Part model, mm, in its own coordinate system. Face numbers are marked on the shaded views. A direction names the side the tool comes from. Round coordinates to 2 decimals unless told otherwise and drop trailing zeros. Loops run counter-clockwise (first coordinate to the right, second up) from the corner with the lowest first, then second, coordinate; pieces in that order, holes last. Notation, with made-up numbers: (57.5, 79) - (97.5, 79) arc R31 cw to (97.5, 109) - close; hole circle Ø1 at (-23, 20.25). An arc over 180 degrees is marked (long way). Put each result on its own line as item: value.
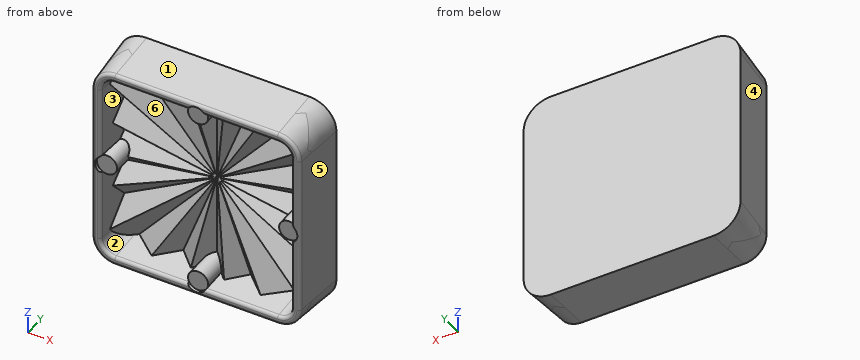
from build123d import *

# Parameters (mm, degrees)
BOSS_EXTRUDE1_DEPTH = 6.35
BOSS_EXTRUDE1_DRAFT = -5
CUT_EXTRUDE3_DEPTH  = 20.05
CIRPATTERN3_COUNT   = 18
BOSS_EXTRUDE3_DEPTH = 6.35
BOSS_EXTRUDE3_DRAFT = -5
FILLET2_R           = 0.381
BOSS_EXTRUDE4_REACH = 20.926
SKETCH8_R           = 1.1811
SKETCH9_R           = 1.1811
CUT_EXTRUDE4_DEPTH  = 19.926409089
CIRPATTERN4_COUNT   = 4


with BuildPart() as part:
    # Sketch1 → Boss-Extrude1 (with draft: the straight prism first)
    with BuildSketch(Plane(origin=(0, 0, 0), x_dir=(1, 0, 0), z_dir=(0, 1, 0))):
        with BuildLine():
            Line((-9.525, -12.7), (9.525, -12.7))
            ThreePointArc((9.525, -12.7), (11.77006403, -11.77006403), (12.7, -9.525))
            Line((12.7, -9.525), (12.7, 9.525))
            ThreePointArc((12.7, 9.525), (11.77006403, 11.77006403), (9.525, 12.7))
            Line((9.525, 12.7), (-9.525, 12.7))
            ThreePointArc((-9.525, 12.7), (-11.77006403, 11.77006403), (-12.7, 9.525))
            Line((-12.7, 9.525), (-12.7, -9.525))
            ThreePointArc((-12.7, -9.525), (-11.77006403, -11.77006403), (-9.525, -12.7))
        make_face()
    extrude(amount=-BOSS_EXTRUDE1_DEPTH)
    # Boss-Extrude1: the draft: its side faces are tilted about the plane it starts from
    boss_extrude1_sides = [part.faces().sort_by_distance(p)[0] for p in [
        (0, -3.175, 12.7),
        (11.77006403, -3.175, 11.77006403),
        (12.7, -3.175, 0),
        (11.77006403, -3.175, -11.77006403),
        (0, -3.175, -12.7),
        (-11.77006403, -3.175, -11.77006403),
        (-12.7, -3.175, 0),
        (-11.77006403, -3.175, 11.77006403),
    ]]
    draft(boss_extrude1_sides, Plane(origin=(0, 0, 0), x_dir=(1, 0, 0), z_dir=(0, 1, 0)), BOSS_EXTRUDE1_DRAFT)

    # Sketch6 → Cut-Extrude3 (cut, through all)
    with BuildSketch(Plane.XY):
        Polygon((0, -2.159), (-7.366, -9.525), (7.366, -9.525), align=None)
    cut_extrude3 = extrude(amount=-CUT_EXTRUDE3_DEPTH, mode=Mode.SUBTRACT)

    # CirPattern3: Cut-Extrude3 ×18 about axis
    cirpattern3_axis = Axis((0, 0, 0), (0, 1, 0))
    for i in range(1, CIRPATTERN3_COUNT):
        add(cut_extrude3.rotate(cirpattern3_axis, i * 360 / CIRPATTERN3_COUNT), mode=Mode.SUBTRACT)


with BuildPart() as boss_extrude3_tool:
    # Sketch7 → Boss-Extrude3 (with draft: the straight prism first)
    with BuildSketch(Plane(origin=(0, 0, 0), x_dir=(1, 0, 0), z_dir=(0, 1, 0))):
        with BuildLine():
            Line((-9.525, -12.7), (9.525, -12.7))
            ThreePointArc((9.525, -12.7), (11.77006403, -11.77006403), (12.7, -9.525))
            Line((12.7, -9.525), (12.7, 9.525))
            ThreePointArc((12.7, 9.525), (11.77006403, 11.77006403), (9.525, 12.7))
            Line((9.525, 12.7), (-9.525, 12.7))
            ThreePointArc((-9.525, 12.7), (-11.77006403, 11.77006403), (-12.7, 9.525))
            Line((-12.7, 9.525), (-12.7, -9.525))
            ThreePointArc((-12.7, -9.525), (-11.77006403, -11.77006403), (-9.525, -12.7))
        make_face()
        with BuildLine():
            Line((-9.525, -10.668), (9.525, -10.668))
            ThreePointArc((9.525, -10.668), (10.333223051, -10.333223051), (10.668, -9.525))
            Line((10.668, -9.525), (10.668, 9.525))
            ThreePointArc((10.668, 9.525), (10.333223051, 10.333223051), (9.525, 10.668))
            Line((9.525, 10.668), (-9.525, 10.668))
            ThreePointArc((-9.525, 10.668), (-10.333223051, 10.333223051), (-10.668, 9.525))
            Line((-10.668, 9.525), (-10.668, -9.525))
            ThreePointArc((-10.668, -9.525), (-10.333223051, -10.333223051), (-9.525, -10.668))
        make_face(mode=Mode.SUBTRACT)
    extrude(amount=-BOSS_EXTRUDE3_DEPTH)
    # Boss-Extrude3: the draft: its side faces are tilted about the plane it starts from
    boss_extrude3_sides = [boss_extrude3_tool.faces().sort_by_distance(p)[0] for p in [
        (0, -3.175, 12.7),
        (11.77006403, -3.175, 11.77006403),
        (12.7, -3.175, 0),
        (11.77006403, -3.175, -11.77006403),
        (0, -3.175, -12.7),
        (-11.77006403, -3.175, -11.77006403),
        (-12.7, -3.175, 0),
        (-11.77006403, -3.175, 11.77006403),
        (-10.333223051, -3.175, 10.333223051),
        (-10.668, -3.175, 0),
        (-10.333223051, -3.175, -10.333223051),
        (0, -3.175, -10.668),
        (10.333223051, -3.175, -10.333223051),
        (10.668, -3.175, 0),
        (10.333223051, -3.175, 10.333223051),
        (0, -3.175, 10.668),
    ]]
    draft(boss_extrude3_sides, Plane(origin=(0, 0, 0), x_dir=(1, 0, 0), z_dir=(0, 1, 0)), BOSS_EXTRUDE3_DRAFT)


with BuildPart() as part_1:
    add(part.part)

    # Boss-Extrude3: add boss_extrude3_tool
    add(boss_extrude3_tool.part)

    # Fillet2
    fillet2_edges = [part_1.edges().sort_by_distance(p)[0] for p in [
        (-11.377228727, -6.35, -11.377228727),
        (-11.377228727, -6.35, 11.377228727),
        (-12.144446987, -6.35, 0),
        (0, -6.35, 12.144446987),
        (11.377228727, -6.35, 11.377228727),
        (12.144446987, -6.35, 0),
        (11.377228727, -6.35, -11.377228727),
        (0, -6.35, -12.144446987),
        (-11.223553013, -6.35, 0),
        (-10.726058354, -6.35, 10.726058354),
        (0, -6.35, 11.223553013),
        (10.726058354, -6.35, 10.726058354),
        (11.223553013, -6.35, 0),
        (10.726058354, -6.35, -10.726058354),
        (0, -6.35, -11.223553013),
        (-10.726058354, -6.35, -10.726058354),
    ]]
    fillet(fillet2_edges, radius=FILLET2_R)

    # Sketch8 → Boss-Extrude4 (add, up to next)
    with BuildSketch(Plane(origin=(0, -5.969, 0), x_dir=(-1, 0, 0), z_dir=(0, -1, 0)), mode=Mode.PRIVATE) as boss_extrude4_sk1:
        with Locations((0, 10.668)):
            Circle(SKETCH8_R)
    boss_extrude4_tool1 = extrude(boss_extrude4_sk1.sketch, amount=-BOSS_EXTRUDE4_REACH, mode=Mode.PRIVATE) - part_1.part
    boss_extrude4 = boss_extrude4_tool1.solids().sort_by_distance((0, -5.969, -10.668))[0]
    add(boss_extrude4)

    # Sketch9 → Cut-Extrude4 (cut, through all)
    with BuildSketch(Plane.XZ.offset(5.969)):
        with Locations((0, -10.668)):
            Circle(SKETCH9_R)
    cut_extrude4 = extrude(amount=CUT_EXTRUDE4_DEPTH, mode=Mode.SUBTRACT)

    # CirPattern4: Boss-Extrude4, Cut-Extrude4; each copy of Boss-Extrude4 runs up to whatever stops it at its own place
    cirpattern4_before = part_1.part  # the part as the pattern finds it: every copy runs up to it
    cirpattern4_boss_extrude4_long = extrude(boss_extrude4_sk1.sketch, amount=-BOSS_EXTRUDE4_REACH, mode=Mode.PRIVATE)
    cirpattern4_boss_extrude4_tool = cirpattern4_boss_extrude4_long.rotate(Axis((0, 0, 0), (0, 1, 0)), 1 * 360 / CIRPATTERN4_COUNT) - cirpattern4_before
    add(cirpattern4_boss_extrude4_tool.solids().sort_by_distance((-10.668, -5.969, 0))[0])
    cirpattern4_boss_extrude4_tool = cirpattern4_boss_extrude4_long.rotate(Axis((0, 0, 0), (0, 1, 0)), 2 * 360 / CIRPATTERN4_COUNT) - cirpattern4_before
    add(cirpattern4_boss_extrude4_tool.solids().sort_by_distance((0, -5.969, 10.668))[0])
    cirpattern4_boss_extrude4_tool = cirpattern4_boss_extrude4_long.rotate(Axis((0, 0, 0), (0, 1, 0)), 3 * 360 / CIRPATTERN4_COUNT) - cirpattern4_before
    add(cirpattern4_boss_extrude4_tool.solids().sort_by_distance((10.668, -5.969, 0))[0])
    add(cut_extrude4.rotate(Axis((0, 0, 0), (0, 1, 0)), 1 * 360 / CIRPATTERN4_COUNT), mode=Mode.SUBTRACT)
    add(cut_extrude4.rotate(Axis((0, 0, 0), (0, 1, 0)), 2 * 360 / CIRPATTERN4_COUNT), mode=Mode.SUBTRACT)
    add(cut_extrude4.rotate(Axis((0, 0, 0), (0, 1, 0)), 3 * 360 / CIRPATTERN4_COUNT), mode=Mode.SUBTRACT)


solid = part_1.part
1. Band-saw the part on A-A (x = -3.5). List the corners of the cut face in (y, z), plus the area to 3 significant figures.
A:
outline: (-6.35, -11.8) arc R0.38 ccw to (-6, -12.17) - (0, -12.7) - (0, 12.7) - (-6, 12.17) arc R0.38 ccw to (-6.35, 11.8) - (-6.35, 11.57) arc R0.38 ccw to (-6, 11.19) - (-2.6, 10.9) - (-2.16, 9.62) - (-3.37, 6.06) - (-2.16, 4.17) - (-2.95, 2.94) - (-2.16, 2.02) - (-2.81, 1.27) - (-2.16, 0.62) - (-2.77, 0) - (-2.16, -0.62) - (-2.81, -1.27) - (-2.16, -2.02) - (-2.95, -2.94) - (-2.16, -4.17) - (-3.37, -6.06) - (-2.16, -9.62) - (-2.6, -10.9) - (-6, -11.19) arc R0.38 ccw to (-6.35, -11.57) - close
area: 75.3 mm²
2. Probe line 1 along X through (y, z) = (-3.5, 8.75); line 2 along Z through (x, y) = (-10, -5.5); line 3 along Z through (x, y) = (8.25, -5). List the from-to ranges inside material, lowest first. Write a range as [from, to].
A:
line 1: x = [-12.39, -9.09], [-5.59, -4.61], [-1.76, -1.34], [1.34, 1.76], [4.61, 5.59], [9.09, 12.39]
line 2: z = [-12.18, -11.08], [-0.97, 0.97], [11.08, 12.18]
line 3: z = [-12.26, -11.11], [11.11, 12.26]
3. Band-saw the part on D-D (x = 8.5). List the corners of the cut face in (y, z) (3 decimals), plus the area to 3 significant figures.
A:
outline: (-6.35, -11.795) arc R0.381 ccw to (-6.002, -12.175) - (0, -12.7) - (0, 12.7) - (-6.002, 12.175) arc R0.381 ccw to (-6.35, 11.795) - (-6.35, 11.573) arc R0.381 ccw to (-6.002, 11.193) - (-2.654, 10.9) - (-2.159, 10.13) - (-4.086, 7.132) - (-2.159, 4.907) - (-3.73, 3.094) - (-2.159, 1.499) - (-3.635, 0) - (-2.159, -1.499) - (-3.73, -3.094) - (-2.159, -4.907) - (-4.086, -7.132) - (-2.159, -10.13) - (-2.654, -10.9) - (-6.002, -11.193) arc R0.381 ccw to (-6.35, -11.573) - close
area: 83.1 mm²
4. Band-saw the part on B-B (z = 5.75). List the corners of the cut face in (x, y).
A:
outline: (-12.7, 0) - (-12.17, -6) arc R0.38 ccw to (-11.8, -6.35) - (-11.57, -6.35) arc R0.38 ccw to (-11.19, -6) - (-10.9, -2.63) - (-9.96, -2.16) - (-6.85, -3.71) - (-4.82, -2.16) - (-3.32, -3.31) - (-2.09, -2.16) - (-1.01, -3.17) - (0, -2.16) - (1.01, -3.17) - (2.09, -2.16) - (3.32, -3.31) - (4.82, -2.16) - (6.85, -3.71) - (9.96, -2.16) - (10.9, -2.63) - (11.19, -6) arc R0.38 ccw to (11.57, -6.35) - (11.8, -6.35) arc R0.38 ccw to (12.17, -6) - (12.7, 0) - close
5. Pin check, flat tips, straight feed: P1, Ø1.5, axis at x = -3.5, y = -2, coming from the -Z side; P2, Ø1, axis at x = -3.5, z = 9.5, coming from the -Y side. Stop position of each tip, or through.
A:
P1: stops at z = -12.59
P2: stops at y = -2.7
6. Band-saw the part on C-C (y = -1.5). List the corners of the cut face in (x, z) (3 decimals), plus the area to 3 significant figures.
A:
outline: (-12.569, -9.525) arc R3.044 ccw to (-9.525, -12.569) - (9.525, -12.569) arc R3.044 ccw to (12.569, -9.525) - (12.569, 9.525) arc R3.044 ccw to (9.525, 12.569) - (-9.525, 12.569) arc R3.044 ccw to (-12.569, 9.525) - close
area: 624 mm²
7. Tool access for the marked faces 5 and 6: list every direction of +Z, -Z, +X, -X, +Y, -Y with a clear straight run to the whole face (end or side of a thin tool).
A:
face 5: +Z, -Z, +X, -Y
face 6: -Y
8. Two-plate mould, pull along Z, no slides. Class the marked faces 1, 2, 3 and 4: pulls with the +Z half, pulls with the -Z half, needs draft (parallel to the pull), parting line crosses it, or undercut.
A:
face 1: pulls with the +Z half
face 2: undercut
face 3: undercut
face 4: needs draft
